```python
from build123d import *

# Parameters (mm, degrees)
SKETCH_1_W                = 42.3
SKETCH_1_H                = 60
EXTRUDE_1_DEPTH           = 42.3
HOLE_WIZARD_3_0_3_1_D     = 3
HOLE_WIZARD_3_0_3_1_DEPTH = 5
CHAMFER_1_SIZE            = 3


with BuildPart() as part:
    # 草图1 → 凸台-拉伸1 (new body)
    with BuildSketch(Plane.XZ.offset(21.15)):
        with Locations((0, 25)):
            Rectangle(SKETCH_1_W, SKETCH_1_H)
    extrude(amount=-EXTRUDE_1_DEPTH)

    # 草图2 → 旋转1 (revolve)
    with BuildSketch(Plane.XZ):
        Polygon((2.5, 79), (0, 79), (0, 55), (11, 55), (11, 57), (2.5, 57), align=None)
    revolve(axis=Axis((0, 0, 79), (0, 0, -1)))

    # Ø3.0 (3) 直径孔1
    with Locations(Plane.XY.offset(55)):
        with Locations((15.5, -15.5), (-15.5, -15.5), (-15.5, 15.5), (15.5, 15.5)):
            Hole(HOLE_WIZARD_3_0_3_1_D / 2, depth=HOLE_WIZARD_3_0_3_1_DEPTH)

    # 倒角1
    chamfer_1_edges = [part.edges().sort_by_distance(p)[0] for p in [
        (-21.15, 21.15, 25),
        (21.15, 21.15, 25),
        (-21.15, -21.15, 25),
        (21.15, -21.15, 25),
    ]]
    chamfer(chamfer_1_edges, length=CHAMFER_1_SIZE)


solid = part.part
```
Verification items for the finished model (mm, model axes). A direction names the side the tool comes from. Round coordinates to 2 decimals unless told otherwise and drop trailing zeros. Loops run counter-clockwise (first coordinate to the right, second up) from the corner with the lowest first, then second, coordinate; pieces in that order, holes last. Notation, with made-up numbers: (2, 3) -> (48, 3) arc R18 ccw to (48, 15) -> close; hole circle Ø10 at (81, 23.5). An arc over 180 degrees is marked (long way). Answer as a JSON object with one key per item and string values.
Q1. Go/stop test with flat-tipped pins: P1, Ø6, axis at x = -3.5, z = 63.5, coming from the +Y side; P2, Ø2.5, axis at x = 15, y = 15.5, coming from the +Z side; P3, Ø1.8, axis at x = -15.5, y = -15.5, coming from the +Z side. Record where each tip stops, or that it passes through.
Data:
{"P1": "stops at y = 2.45", "P2": "stops at z = 55", "P3": "stops at z = 50"}
Q2. Access from +Z, -Z, +X, -X, +Y, -Y to the whole of each face (thin tool, end or side, straight path). Record for faces 5 (the flat face through (-10, -10, 55)), 6 (the flat face through (0, -21.15, 25)).
Data:
{"face 5": "+Z", "face 6": "+Z, -Z, +X, -X, -Y"}
Q3. Section check A-A (z = 52.5). Record the boundary of the cut face in (x, y), then the cut area to 3 significant figures.
Data:
{"outline": "(-21.15, -18.15) -> (-18.15, -21.15) -> (18.15, -21.15) -> (21.15, -18.15) -> (21.15, 18.15) -> (18.15, 21.15) -> (-18.15, 21.15) -> (-21.15, 18.15) -> close; hole circle Ø3 at (-15.5, -15.5); hole circle Ø3 at (-15.5, 15.5); hole circle Ø3 at (15.5, -15.5); hole circle Ø3 at (15.5, 15.5)", "area": "1,740 mm2"}
Q4. Scan lines: line 1 (Y direction, x = -15.5, z = 51.4); line 2 (X direction, y = -15, z = 51); line 3 (Z direction, x = 11, y = 5). Record each from-to range of solid material in increasing order. Write a range as from..to.
Data:
{"line 1": "y = -21.15..-17, -14..14, 17..21.15", "line 2": "x = -21.15..-16.91, -14.09..14.09, 16.91..21.15", "line 3": "z = -5..55"}
Q5. Section check B-B (y = 0). Record the boundary of the cut face in (x, z).
Data:
{"outline": "(-21.15, -5) -> (21.15, -5) -> (21.15, 55) -> (11, 55) -> (11, 57) -> (2.5, 57) -> (2.5, 79) -> (-2.5, 79) -> (-2.5, 57) -> (-11, 57) -> (-11, 55) -> (-21.15, 55) -> close"}
Q6. Draft check along Y on faces 1 (the flat face through (21.15, 0, 25)), 2 (the flat face through (19.7, 19.6, 24.6)), 3 (the flat face through (16, 16, 50)), 4 (the cylindrical face through (-14, 15.57, 52.46)). Enter one of: pulls with the +Y half, pulls with the -Y half, needs draft (parallel to the pull), parting line crosses it, or undercut.
Data:
{"face 1": "needs draft", "face 2": "pulls with the +Y half", "face 3": "undercut", "face 4": "undercut"}
Q7. Section check D-D (y = -8). Record the boundary of the cut face in (x, z), then the cut area to 3 significant figures.
Data:
{"outline": "(-21.15, -5) -> (21.15, -5) -> (21.15, 55) -> (7.55, 55) -> (7.55, 57) -> (-7.55, 57) -> (-7.55, 55) -> (-21.15, 55) -> close", "area": "2,570 mm2"}
Q8. Section check C-C (x = 15.5). Record the boundary of the cut face in (y, z), then the cut area to 3 significant figures.
Data:
{"outline": "(-21.15, -5) -> (21.15, -5) -> (21.15, 55) -> (17, 55) -> (17, 50) -> (14, 50) -> (14, 55) -> (-14, 55) -> (-14, 50) -> (-17, 50) -> (-17, 55) -> (-21.15, 55) -> close", "area": "2,510 mm2"}
